Design review of the part built by this model. Coordinates are the model's own, in mm. Round coordinates to 2 decimals unless told otherwise and drop trailing zeros. Write each loop counter-clockwise with the first axis right and the second up, starting at its lowest first coordinate (ties: lowest second). Pieces come first, ordered by that corner, then holes. Notation, with made-up numbers: (22, -24.5) -> (28, -24.5) arc R27 cw to (28, -6.5) -> close; hole circle Ø10 at (5, 17.25). An arc over 180 degrees is marked (long way). Write item = value, one per line. Start each with the question number.
Item 1: To check wall thickness, follow L1, parallel to Z at x = 54.5, y = 0.65; L2, parallel to X at y = 3, z = -21; L3, parallel to X at y = 0.75, z = -102.5 (3 decimals). State the ranges of each line that lie inside material, in increasing order.
Item 2: Add section C-C, the plane y = 1.75. State how many separate pieces and enclosed holes the cut face has, then the cut area to 3 significant figures.
Item 3: For pin 1 Ø1.6 at (y, z) = (1, -71) entering from +X; pin 2 Ø1.5 at (y, z) = (1.5, -14.5) entering from -X; pin 3 Ø1 at (x, y) = (-102.5, 2) entering from -Z (3 decimals), all flat-tipped, find the tip position at first contact; note any pin that passes through.
Item 4: Add section D-D, the plane z = 52.5. State the section outline as (x, y) points (3 decimals).
Item 5: Add section A-A, the plane z = -23.5. State the section outline as (x, y) points (3 decimals), then the cut area to 3 significant figures.
Item 6: Add section B-B, the plane x = 26. State the section outline as (y, z) points (3 decimals).
from build123d import *

# Parameters (mm, degrees)
SKETCH1_W           = 3.175
SKETCH1_H           = 15
BOSS_EXTRUDE1_DEPTH = 3.175


with BuildPart() as part:
    # Sketch1 → Boss-Extrude1 (new body)
    with BuildSketch(Plane(origin=(0, 0, 0), x_dir=(1, 0, 0), z_dir=(0, 1, 0))):
        with BuildLine():
            Line((-55, 0), (55, 0))
            Line((55, 0), (55, 57.88))
            Line((55, 57.88), (51.825, 57.88))
            Line((51.825, 57.88), (51.825, 61.055))
            Line((51.825, 61.055), (48.65, 61.055))
            Line((48.65, 61.055), (48.65, 57.88))
            ThreePointArc((48.65, 57.88), (43.65, 62.88), (48.65, 67.88))
            Line((48.65, 67.88), (55, 67.88))
            Line((55, 67.88), (55, 77.88))
            Line((55, 77.88), (48.65, 77.88))
            ThreePointArc((48.65, 77.88), (43.65, 82.88), (48.65, 87.88))
            Line((48.65, 87.88), (48.65, 84.705))
            Line((48.65, 84.705), (51.825, 84.705))
            Line((51.825, 84.705), (51.825, 87.88))
            Line((51.825, 87.88), (55, 87.88))
            Line((55, 87.88), (55, 112.88))
            Line((55, 112.88), (76.2, 112.88))
            Line((76.2, 112.88), (86.2, 112.88))
            Line((86.2, 112.88), (97.2, 112.88))
            Line((97.2, 112.88), (97.2, 87.88))
            Line((97.2, 87.88), (100.375, 87.88))
            Line((100.375, 87.88), (100.375, 84.705))
            Line((100.375, 84.705), (103.55, 84.705))
            Line((103.55, 84.705), (103.55, 87.88))
            ThreePointArc((103.55, 87.88), (108.55, 82.88), (103.55, 77.88))
            Line((103.55, 77.88), (97.2, 77.88))
            Line((97.2, 77.88), (97.2, 67.88))
            Line((97.2, 67.88), (103.55, 67.88))
            ThreePointArc((103.55, 67.88), (108.55, 62.88), (103.55, 57.88))
            Line((103.55, 57.88), (103.55, 61.055))
            Line((103.55, 61.055), (100.375, 61.055))
            Line((100.375, 61.055), (100.375, 57.88))
            Line((100.375, 57.88), (97.2, 57.88))
            Line((97.2, 57.88), (97.2, 11))
            ThreePointArc((97.2, 11), (89.421825407, 7.778174593), (86.2, 0))
            Line((86.2, 0), (86.2, -102.88))
            Line((86.2, -102.88), (86.2, -112.88))
            Line((86.2, -112.88), (76.2, -112.88))
            Line((76.2, -112.88), (-76.2, -112.88))
            Line((-76.2, -112.88), (-86.2, -112.88))
            Line((-86.2, -112.88), (-86.2, -102.88))
            Line((-86.2, -102.88), (-86.2, 0))
            ThreePointArc((-86.2, 0), (-89.421825407, 7.778174593), (-97.2, 11))
            Line((-97.2, 11), (-97.2, 57.88))
            Line((-97.2, 57.88), (-100.375, 57.88))
            Line((-100.375, 57.88), (-100.375, 61.055))
            Line((-100.375, 61.055), (-103.55, 61.055))
            Line((-103.55, 61.055), (-103.55, 57.88))
            ThreePointArc((-103.55, 57.88), (-108.55, 62.88), (-103.55, 67.88))
            Line((-103.55, 67.88), (-97.2, 67.88))
            Line((-97.2, 67.88), (-97.2, 77.88))
            Line((-97.2, 77.88), (-103.55, 77.88))
            ThreePointArc((-103.55, 77.88), (-108.55, 82.88), (-103.55, 87.88))
            Line((-103.55, 87.88), (-103.55, 84.705))
            Line((-103.55, 84.705), (-100.375, 84.705))
            Line((-100.375, 84.705), (-100.375, 87.88))
            Line((-100.375, 87.88), (-97.2, 87.88))
            Line((-97.2, 87.88), (-97.2, 112.88))
            Line((-97.2, 112.88), (-86.2, 112.88))
            Line((-86.2, 112.88), (-76.2, 112.88))
            Line((-76.2, 112.88), (-55, 112.88))
            Line((-55, 112.88), (-55, 87.88))
            Line((-55, 87.88), (-51.825, 87.88))
            Line((-51.825, 87.88), (-51.825, 84.705))
            Line((-51.825, 84.705), (-48.65, 84.705))
            Line((-48.65, 84.705), (-48.65, 87.88))
            ThreePointArc((-48.65, 87.88), (-43.65, 82.88), (-48.65, 77.88))
            Line((-48.65, 77.88), (-55, 77.88))
            Line((-55, 77.88), (-55, 67.88))
            Line((-55, 67.88), (-48.65, 67.88))
            ThreePointArc((-48.65, 67.88), (-43.65, 62.88), (-48.65, 57.88))
            Line((-48.65, 57.88), (-48.65, 61.055))
            Line((-48.65, 61.055), (-51.825, 61.055))
            Line((-51.825, 61.055), (-51.825, 57.88))
            Line((-51.825, 57.88), (-55, 57.88))
            Line((-55, 57.88), (-55, 0))
        make_face()
        with Locations((74.6125, 95.38)):
            Rectangle(SKETCH1_W, SKETCH1_H, mode=Mode.SUBTRACT)
        with Locations((-74.6125, 95.38)):
            Rectangle(SKETCH1_W, SKETCH1_H, mode=Mode.SUBTRACT)
        with Locations((-74.6125, -95.38)):
            Rectangle(SKETCH1_W, SKETCH1_H, mode=Mode.SUBTRACT)
        with Locations((74.6125, -95.38)):
            Rectangle(SKETCH1_W, SKETCH1_H, mode=Mode.SUBTRACT)
    extrude(amount=BOSS_EXTRUDE1_DEPTH)


solid = part.part
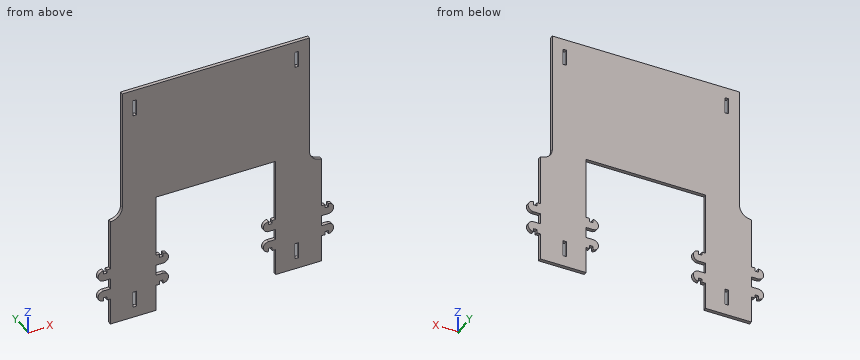
Result set:
q1.L1 = -87.88 to -77.88, -67.88 to -57.88, 0 to 112.88
q1.L2 = -97.2 to -55, 55 to 97.2
q1.L3 = -97.2 to -76.2, -73.025 to -55, 55 to 73.025, 76.2 to 97.2
q2.separate_pieces = 1
q2.enclosed_holes = 4
q2.area = 29,300 mm²
q3.pin_1 = 97.2
q3.pin_2 = -97.2
q3.pin_3 = -84.705
q4.outline = (-86.2, 0) -> (86.2, 0) -> (86.2, 3.175) -> (-86.2, 3.175) -> close
q5.outline = (-97.2, 0) -> (-55, 0) -> (-55, 3.175) -> (-97.2, 3.175) -> close; (55, 0) -> (97.2, 0) -> (97.2, 3.175) -> (55, 3.175) -> close
q5.area = 268 mm²
q6.outline = (0, 0) -> (3.175, 0) -> (3.175, 112.88) -> (0, 112.88) -> close
